Read the model definition and answer for the solid it produces. Units are mm, in the model's axes. A direction names the side the tool comes from. Coordinates: 2 decimals unless noted, no trailing zeros. Write each loop counter-clockwise with the first axis right and the second up, starting at its lowest first coordinate (ties: lowest second). Pieces come first, ordered by that corner, then holes. Notation, with made-up numbers: (60.25, -7) -> (73.25, -7) arc R36 cw to (73.25, 31) -> close; hole circle Ø4 at (8.5, 13.5). An arc over 180 degrees is marked (long way). Answer in a Markdown table with one row per item. Add a question column.
Item 1: Straight lines are drawn through the part: line 1 (Z direction, x = -8.75, y = -2); line 2 (Y direction, x = -0.5, z = -21.75); line 3 (X direction, y = -3, z = -4). For each, find the intervals that lie inside material, in ascending order. Write a range as from..to.
Item 2: Which of the six approach directions +Z, -Z, +X, -X, +Y, -Y give full straight-line access (tool end or side, diameter ignored) to faces 4 (the face through (6.466, -2.681, -12.62)), 5 (the face through (-1.08, -4.88, -14.62)), 6 (the face through (2, 6, -25))?
Item 3: Section C-C on z = -9.75 is taken. Write down the section's boundary in (x, y).
Item 4: Given pin 1 Ø12 at (y, z) = (3, -14.5) entering from -X; pin 2 Ø4 at (y, z) = (0, -17) entering from +X; pin 3 Ø3.5 at (x, y) = (-0.5, 0) entering from -Z, each flat-ended and moving along its own axis, determine where each tip first touches the part or whether it passes through.
Item 5: For a pull along X with two mould halves and no side action, classify faces 1 (the face through (3.5, 1.1, -0.17)), 2 (the face through (2, 0, 0)), 3 (the face through (-1.5, 0.07, -0.99)) as +X half, -X half, draft (parallel to the pull), parting line (faces both ways), or undercut.
```python
from build123d import *

# Parameters (mm, degrees)
F0_R     = 7
F0_R_2   = 1.5
F1_DEPTH = 25
F2_T     = -2
F3_DEPTH = 25
F4_R     = 10
F4_R_2   = 7
F5_DEPTH = 2
F6_SIZE  = 1
F7_SIZE  = 3.49999


# Not quite as in the source:
# - a fillet or chamfer is up to 0.001 mm smaller than in the source, because OpenCascade refuses the exact size


with BuildPart() as f1:
    # F0 (on Top) → F1 (new body)
    with BuildSketch(Plane.XY):
        Circle(F0_R)
        Circle(F0_R_2, mode=Mode.SUBTRACT)
        Circle(F0_R_2)
    extrude(amount=-F1_DEPTH)

    # F2
    f2_openings = [f1.faces().sort_by_distance(p)[0] for p in [
        (0, 0, -25),
    ]]
    offset(amount=F2_T, openings=f2_openings)

    # F0 (on Top) → F3 (cut)
    with BuildSketch(Plane.XY):
        Circle(F0_R_2)
    extrude(amount=-F3_DEPTH, mode=Mode.SUBTRACT)

    # F4 (on face) → F5 (join)
    with BuildSketch(Plane(origin=(0, 0, -25), x_dir=(1, 0, 0), z_dir=(0, 0, -1))):
        Circle(F4_R)
        Circle(F4_R_2, mode=Mode.SUBTRACT)
    extrude(amount=-F5_DEPTH)

    # F6
    f6_edges = [f1.edges().sort_by_distance(p)[0] for p in [
        (-7, 0, -23),
        (-5, 0, -25),
        (-10, 0, -25),
    ]]
    chamfer(f6_edges, length=F6_SIZE)

    # F7 (size 3.5 in the source; OpenCascade refuses exactly that, so slightly less here)
    f7_edges = [f1.edges().sort_by_distance(p)[0] for p in [
        (-7, 0, 0),
        (-5, 0, -2),
    ]]
    chamfer(f7_edges, length=F7_SIZE)


solid = f1.part
```
Results below:
| question | item | result |
|---|---|---|
| 1 | line 1 | z = -25..-23 |
| 1 | line 2 | y = -6.98..-4.97, 4.97..6.98 |
| 1 | line 3 | x = -6.32..-1.8, 1.8..6.32 |
| 2 | face 4 | +Z |
| 2 | face 5 | -Z |
| 2 | face 6 | -Z, +X, -X, +Y, -Y |
| 3 | outline | circle Ø14 at (0, 0); hole circle Ø10 at (0, 0) |
| 4 | pin 1 | stops at x = -7 |
| 4 | pin 2 | stops at x = 7 |
| 4 | pin 3 | stops at z = -2.75 |
| 5 | face 1 | parting line |
| 5 | face 2 | draft |
| 5 | face 3 | undercut |
